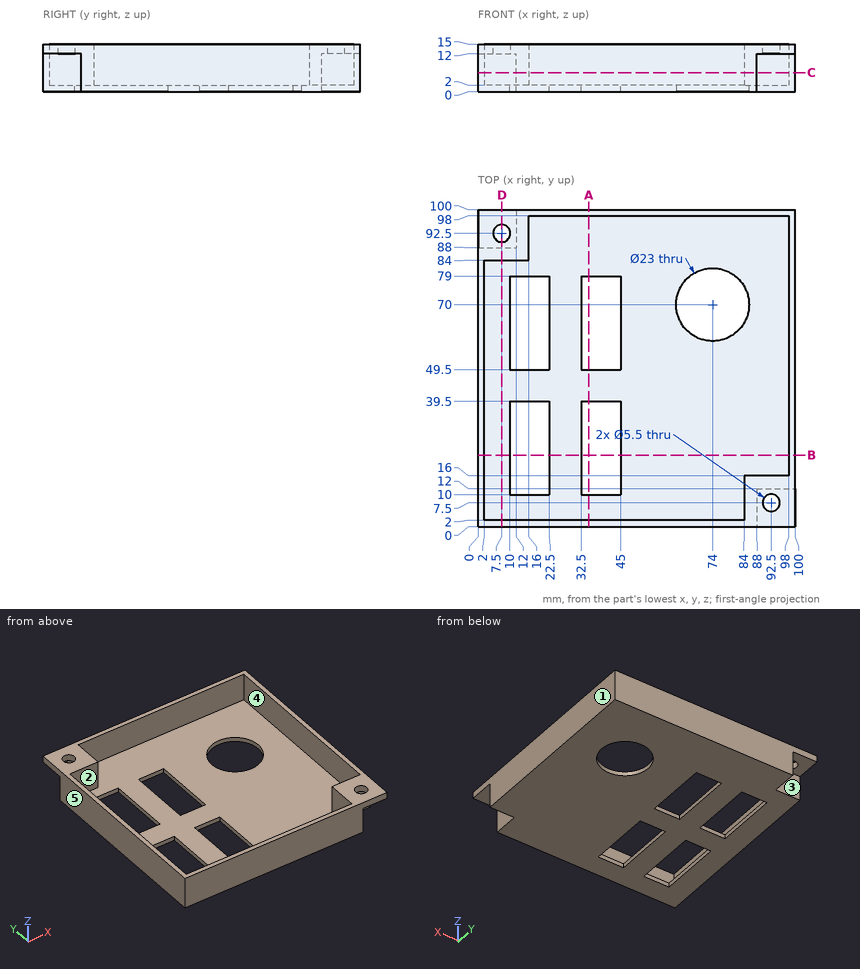
Geometry: see drawing. Coordinates: mm, zero at the bounding-box minimum. A direction names the side the tool comes from. Round coordinates to 2 decimals unless told otherwise and drop trailing zeros. Loops run counter-clockwise (first coordinate to the right, second up) from the corner with the lowest first, then second, coordinate; pieces in that order, holes last. Notation, with made-up numbers: (-11, 42.25) - (15, 42.25) arc R28 ccw to (15, 69.25) - close; hole circle Ø8 at (48.5, 41.25). An arc over 180 degrees is marked (long way). One line per item, written item: value. Start each with the question number.
(1) Ray query, line 1 (Y direction, x = 7.5, z = 13.25); line 2 (Y direction, x = 87.5, z = 8.5); line 3 (X direction, y = 70, z = 1.3). Return the intervals inside material, ascending. Write a range as [from, to].
(2) Section A-A, the plane x = 35. Return loops of the section in (y, z), plus the area to 3 significant figures.
(3) Contact query for flat-ended pins moving along their axis: P1, Ø2, axis at x = 27.5, y = 21, coming from the +Z side; P2, Ø3.5, axis at x = 95, y = 5, coming from the -Z side. Output: stop coordinate, or through.
(4) Section C-C, the plane z = 6. Return loops of the section in (x, y), plus the area to 3 significant figures.
(5) Access query for the marked faces 1 and 2. Directions: +Z, -Z, +X, -X, +Y, -Y. A direction counts if a zero-diameter tool reaches every point of the face in a straight line with its end or side. Return the directions, or none.
(6) Draft query along X for the marked faces 3, 4 and 5. Return one class per face: +X half, -X half, draft (parallel to the pull), parting line (faces both ways), or undercut.
(7) Section D-D, the plane x = 7.5. Return loops of the section in (y, z), plus the area to 4 significant figures.
(8) Section B-B, the plane y = 22.5. Return loops of the section in (x, z), plus the area to 3 significant figures.
Results below:
1. line 1: [0, 2], [84, 89.75], [95.25, 100]
1. line 2: [0, 16], [98, 100]
1. line 3: [0, 10], [22.5, 32.5], [45, 62.5], [85.5, 100]
2. outline: (0, 0) - (10, 0) - (10, 2) - (2, 2) - (2, 15) - (0, 15) - close; (39.5, 0) - (49.5, 0) - (49.5, 2) - (39.5, 2) - close; (79, 0) - (100, 0) - (100, 15) - (98, 15) - (98, 2) - (79, 2) - close
2. area: 134 mm^2
3. P1: z = 2
3. P2: z = 12
4. outline: (0, 0) - (88, 0) - (88, 12) - (100, 12) - (100, 100) - (12, 100) - (12, 88) - (0, 88) - close; hole (2, 2) - (84, 2) - (84, 16) - (98, 16) - (98, 98) - (16, 98) - (16, 84) - (2, 84) - close
4. area: 888 mm^2
5. face 1: +Z, -Z, +X, +Y, -Y
5. face 2: +Z
6. face 3: draft
6. face 4: undercut
6. face 5: -X half
7. outline: (0, 0) - (88, 0) - (88, 12) - (89.75, 12) - (89.75, 15) - (84, 15) - (84, 2) - (2, 2) - (2, 15) - (0, 15) - close; (95.25, 12) - (100, 12) - (100, 15) - (95.25, 15) - close
7. area: 273.5 mm^2
8. outline: (0, 0) - (10, 0) - (10, 2) - (2, 2) - (2, 15) - (0, 15) - close; (22.5, 0) - (32.5, 0) - (32.5, 2) - (22.5, 2) - close; (45, 0) - (100, 0) - (100, 15) - (98, 15) - (98, 2) - (45, 2) - close
8. area: 202 mm^2
